Job drawing, mm, ordinate dimensions from the low corner. One solid piece. Round coordinates to 2 decimals unless told otherwise and drop trailing zeros. Loops run counter-clockwise (first coordinate to the right, second up) from the corner with the lowest first, then second, coordinate; pieces in that order, holes last.
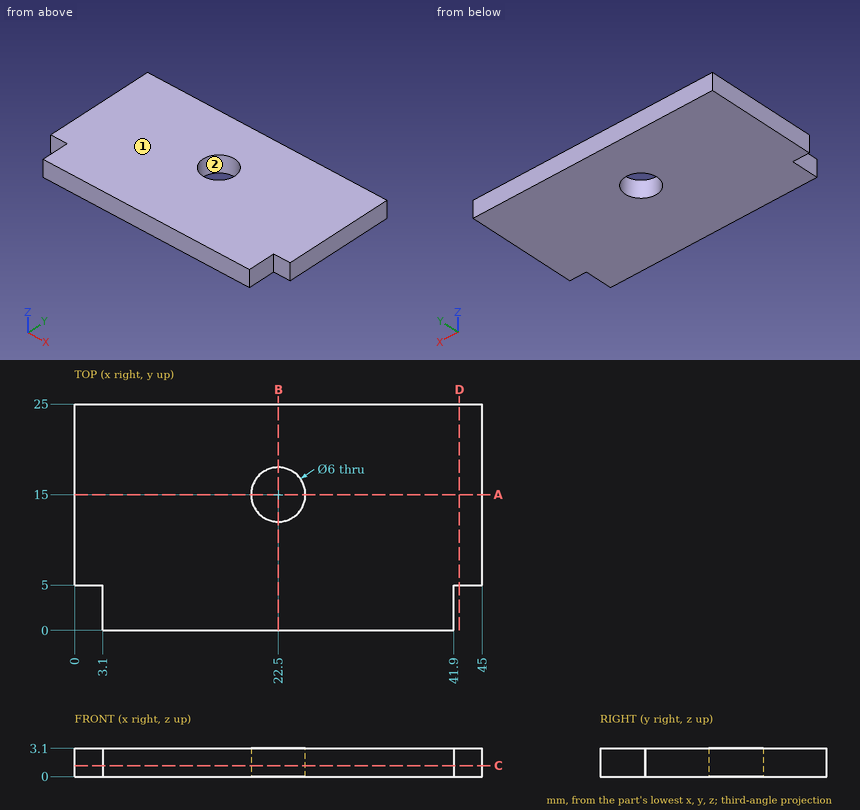
1) Slice it at C-C, the plane z = 1.2. Give the cut face in (x, y), then the cut area to 3 significant figures.
Values:
outline: (0, 5) - (3.1, 5) - (3.1, 0) - (41.9, 0) - (41.9, 5) - (45, 5) - (45, 25) - (0, 25) - close; hole circle Ø6 at (22.5, 15)
area: 1,070 mm2
2) Wall check: line 1 along Y through (x, z) = (22.5, 1.6); line 2 along X through (y, z) = (4.25, 2.05); line 3 along Y through (x, z) = (21.5, 2.55). Give the ranges that are in metal, low to high.
Values:
line 1: y = 0 to 12, 18 to 25
line 2: x = 3.1 to 41.9
line 3: y = 0 to 12.17, 17.83 to 25
3) Slice it at A-A, the plane y = 15. Give the cut face in (x, z).
Values:
outline: (0, 0) - (19.5, 0) - (19.5, 3.1) - (0, 3.1) - close; (25.5, 0) - (45, 0) - (45, 3.1) - (25.5, 3.1) - close
4) Slice it at D-D, the plane x = 42.5. Give the cut face in (y, z), then the cut area to 3 significant figures.
Values:
outline: (5, 0) - (25, 0) - (25, 3.1) - (5, 3.1) - close
area: 62.0 mm2
5) Drop a flat-ended pin along its axis: pin 1 Ø2 at (x, y) = (24, 15) entering from +Z. Give the stop position or say it passes through.
Values:
pin 1: passes through
6) Slice it at B-B, the plane x = 22.5. Give the cut face in (y, z).
Values:
outline: (0, 0) - (12, 0) - (12, 3.1) - (0, 3.1) - close; (18, 0) - (25, 0) - (25, 3.1) - (18, 3.1) - close
7) Mould opens along X. For the marked faces 1 and 2 say: released by +X, released by -X, zero draft, split by the parting line, or undercut.
Values:
face 1: zero draft
face 2: undercut
